The model under review builds one solid part; all positions refer to its coordinate system, in mm. A direction names the side the tool comes from. Coordinates: 2 decimals unless noted, no trailing zeros. Order: outer loops, then holes, each group sorted by start corner. A loop starts at its lowest first (then second) coordinate and runs counter-clockwise, first axis right, second up. Notation, with made-up numbers: (1.5, -22) -> (14.5, -22) arc R12 ccw to (14.5, -8) -> close; hole circle Ø8 at (58, -0.75). An arc over 180 degrees is marked (long way). Answer as CSV lines item,"result". Start each with the question number.
from build123d import *

# Parameters (mm, degrees)
SKETCH3_W                       = 56
SKETCH3_H                       = 3
SKETCH3_W_2                     = 3
SKETCH3_H_2                     = 56
CUT_EXTRUDE1_DEPTH              = 1
BOSS_EXTRUDE1_REACH             = 130.862
SKETCH4_W                       = 31
SKETCH4_H                       = 21
BOSS_EXTRUDE1_DIRECTION_2_REACH = 130.862
CIRPATTERN1_COUNT               = 8


with BuildPart() as part:
    # Sketch2 → Revolve1 (revolve)
    with BuildSketch(Plane(origin=(0, 0, 0), x_dir=(0, 0, -1), z_dir=(1, 0, 0))):
        Polygon((-90.5, 4.121863799), (-57, 4.121863799), (-57, 6.121863799), (-57, 24.121863799), (-59, 24.121863799), (-59, 9.121863799), (-90.5, 9.121863799), align=None)
    revolve(axis=Axis((0, 80.23297491, 0), (0, -1, 0)))

    # Sketch3 → Cut-Extrude1 (cut)
    with BuildSketch(Plane(origin=(0, 9.121863799, 0), x_dir=(1, 0, 0), z_dir=(0, 1, 0))):
        with Locations((-86.980929121, 0)):
            Rectangle(SKETCH3_W, SKETCH3_H)
        Polygon((-82.985966376, 81.743596048), (-80.864646033, 83.864916391), (-41.266666286, 44.266936645), (-43.38798663, 42.145616301), align=None)
        with Locations((0, 89.981852183)):
            Rectangle(SKETCH3_W_2, SKETCH3_H_2)
        Polygon((81.743596048, 85.986889438), (83.864916391, 83.865569094), (44.266936645, 44.267589348), (42.145616301, 46.388909691), align=None)
        with Locations((89.981852183, 3.000923062)):
            Rectangle(SKETCH3_W, SKETCH3_H)
        Polygon((85.986889438, -78.742672986), (83.865569094, -80.86399333), (44.267589348, -41.266013583), (46.388909691, -39.14469324), align=None)
        with Locations((3.000923062, -86.980929121)):
            Rectangle(SKETCH3_W_2, SKETCH3_H_2)
        Polygon((-78.742672986, -82.985966376), (-80.86399333, -80.864646033), (-41.266013583, -41.266666286), (-39.14469324, -43.38798663), align=None)
    extrude(amount=-CUT_EXTRUDE1_DEPTH, mode=Mode.SUBTRACT)

    # Boss-Extrude1: up to this face of the body (flat: up to its plane)
    boss_extrude1_end = Plane(part.part.faces().sort_by_distance((0, 24.121863799, -58.668772004))[0])
    # Sketch4 → Boss-Extrude1 (add, up to the picked face)
    with BuildSketch(Plane(origin=(0, 9.121863799, 0), x_dir=(1, 0, 0), z_dir=(0, 1, 0)), mode=Mode.PRIVATE) as boss_extrude1_sk1:
        with BuildLine():
            Line((18.5, 86.03), (18.5, 59.03))
            Line((18.5, 59.03), (18.5, 55.707696119))
            ThreePointArc((18.5, 55.707696119), (0, 58.209424556), (-18.5, 55.707696119))
            Line((-18.5, 55.707696119), (-18.5, 59.03))
            Line((-18.5, 59.03), (-18.5, 86.03))
            Line((-18.5, 86.03), (18.5, 86.03))
        make_face()
        with Locations((0, 72.53)):
            Rectangle(SKETCH4_W, SKETCH4_H, mode=Mode.SUBTRACT)
    boss_extrude1_tool1 = split(extrude(boss_extrude1_sk1.sketch, amount=BOSS_EXTRUDE1_REACH, mode=Mode.PRIVATE), bisect_by=boss_extrude1_end, keep=Keep.BOTH, mode=Mode.PRIVATE)
    boss_extrude1 = boss_extrude1_tool1.solids().sort_by(Axis((18.021623, 9.121864, -72.53), (0, 1, 0)))[0]
    add(boss_extrude1)

    # Boss-Extrude1 direction 2: up to this face of the body (flat: up to its plane)
    boss_extrude1_direction_2_end = Plane(part.part.faces().sort_by_distance((-52.938409817, 8.121863799, -53.817117102))[0])
    # Sketch4 → Boss-Extrude1 direction 2 (add, up to the picked face)
    with BuildSketch(Plane(origin=(0, 9.121863799, 0), x_dir=(1, 0, 0), z_dir=(0, 1, 0)), mode=Mode.PRIVATE) as boss_extrude1_direction_2_sk1:
        with BuildLine():
            Line((18.5, 86.03), (18.5, 59.03))
            Line((18.5, 59.03), (18.5, 55.707696119))
            ThreePointArc((18.5, 55.707696119), (0, 58.209424556), (-18.5, 55.707696119))
            Line((-18.5, 55.707696119), (-18.5, 59.03))
            Line((-18.5, 59.03), (-18.5, 86.03))
            Line((-18.5, 86.03), (18.5, 86.03))
        make_face()
        with Locations((0, 72.53)):
            Rectangle(SKETCH4_W, SKETCH4_H, mode=Mode.SUBTRACT)
    boss_extrude1_direction_2_tool1 = split(extrude(boss_extrude1_direction_2_sk1.sketch, amount=-BOSS_EXTRUDE1_DIRECTION_2_REACH, mode=Mode.PRIVATE), bisect_by=boss_extrude1_direction_2_end, keep=Keep.BOTH, mode=Mode.PRIVATE)
    boss_extrude1_direction_2 = boss_extrude1_direction_2_tool1.solids().sort_by(Axis((18.021623, 9.121864, -72.53), (0, -1, 0)))[0]
    add(boss_extrude1_direction_2)

    # CirPattern1: Boss-Extrude1, Boss-Extrude1 direction 2 ×8 about axis
    cirpattern1_axis = Axis((0, 0, 0), (0, 1, 0))
    add([boss_extrude1.rotate(cirpattern1_axis, i * 360 / CIRPATTERN1_COUNT) for i in range(1, CIRPATTERN1_COUNT)])
    add([boss_extrude1_direction_2.rotate(cirpattern1_axis, i * 360 / CIRPATTERN1_COUNT) for i in range(1, CIRPATTERN1_COUNT)])


solid = part.part
1) Consider section C-C (y = 11.5). Count the separate pieces of the cut face and the enclosed holes in it, plus the area to 3 significant figures.
2) Tool access review of faces 4 (the face through (63.157, 16.517, 36.994)), 5 (the face through (-51, 8.122, -52)), 6 (the face through (-71, 17, -18.5)): name each direction out of +Z, -Z, +X, -X, +Y, -Y from which nothing blocks a thin tool from reaching the whole face with its end or side.
3) Insertion check: pin 1 Ø3 at (x, y) = (68.5, 8) entering from +Z; pin 2 Ø7.5 at (x, y) = (69, 19.5) entering from -Z; pin 3 Ø4.5 at (x, y) = (70, 15.5) entering from +Z; pin 4 Ø11.5 at (x, z) = (-46, -76) entering from +Y. Each pin has a flat end and moves straight along its axis. Give the tip position at first contact, or say it passes through.
4) Consider section A-A (x = -39). Give the boundary of the cut face in (y, z), plus the area to 3 significant figures.
5) Mouldability with a two-part tool opening along Z and no side actions: class faces 1 (the face through (-27.18, 6.59, 86.32)), 2 (the face through (0, 16, 86.03)), 3 (the face through (54.532, 16.517, 22.522)) as released by +Z, released by -Z, zero draft, split by the parting line, or undercut.
6) Consider section B-B (z = 76). Give the boundary of the cut face in (x, y), plus the area to 3 significant figures.
7) Consider section D-D (x = 76). Give the boundary of the cut face in (y, z), plus the area to 3 significant figures.
8) Wall thickness on L1, parallel to X at y = 18.5, z = 0; L2, parallel to Z at x = 60, y = 12.75: over which ranges is each line inside the solid? List them lowest first. Write a range as [from, to].
Result:
1,separate pieces,"1"
1,enclosed holes,"9"
1,area,"3,810 mm2"
2,face 4,"+X, +Y"
2,face 5,"+Y"
2,face 6,"-X, +Y"
3,pin 1,"z = 60.84"
3,pin 2,"z = -56.41"
3,pin 3,"z = 53.91"
3,pin 4,"y = 24.12"
4,outline,"(4.12, -81.67) -> (9.12, -81.67) -> (9.12, -65.16) -> (24.12, -65.16) -> (24.12, -60.92) -> (9.12, -60.92) -> (9.12, -48.72) -> (24.12, -48.72) -> (24.12, -41.57) -> (4.12, -41.57) -> close; (4.12, 41.57) -> (24.12, 41.57) -> (24.12, 48.72) -> (9.12, 48.72) -> (9.12, 60.92) -> (24.12, 60.92) -> (24.12, 65.16) -> (9.12, 65.16) -> (9.12, 81.67) -> (4.12, 81.67) -> close"
4,area,"743 mm2"
5,face 1,"split by the parting line"
5,face 2,"released by +Z"
5,face 3,"undercut"
6,outline,"(-49.14, 4.12) -> (49.14, 4.12) -> (49.14, 9.12) -> (18.5, 9.12) -> (18.5, 24.12) -> (15.5, 24.12) -> (15.5, 9.12) -> (4.5, 9.12) -> (4.5, 8.12) -> (1.5, 8.12) -> (1.5, 9.12) -> (-15.5, 9.12) -> (-15.5, 24.12) -> (-18.5, 24.12) -> (-18.5, 9.12) -> (-49.14, 9.12) -> close"
6,area,"578 mm2"
7,outline,"(4.12, -49.14) -> (9.12, -49.14) -> (9.12, -18.5) -> (24.12, -18.5) -> (24.12, -15.5) -> (9.12, -15.5) -> (9.12, -4.5) -> (8.12, -4.5) -> (8.12, -1.5) -> (9.12, -1.5) -> (9.12, 15.5) -> (24.12, 15.5) -> (24.12, 18.5) -> (9.12, 18.5) -> (9.12, 49.14) -> (4.12, 49.14) -> close"
7,area,"578 mm2"
8,L1,"[-86.03, -83.03], [-62.03, -57], [57, 62.03], [83.03, 86.03]"
8,L2,"[-61.66, -57.42], [-38.08, -33.84], [-18.5, 18.5], [33.84, 38.08], [57.42, 61.66]"
